Input: part model. Units: mm. Frame: model coordinates. A direction names the side the tool comes from. Round coordinates to 2 decimals unless told otherwise and drop trailing zeros. Order: outer loops, then holes, each group sorted by start corner. A loop starts at its lowest first (then second) coordinate and runs counter-clockwise, first axis right, second up.
Item 1: Cut plane A-A on z = 0. Give the number of separate pieces and of enclosed holes in the cut face, then the cut area to 3 significant figures.
Item 2: Cut plane C-C on x = 155. Output: boundary loops of the cut face in (y, z).
Item 3: Cut plane B-B on y = 0.1. Output: boundary loops of the cut face in (x, z), then the cut area to 3 significant figures.
Item 4: Cut plane D-D on x = 27. Output: boundary loops of the cut face in (y, z), then the cut area to 3 significant figures.
Item 5: Reachability of faces 1 (the flat face through (196.5, -2, 0)), 2 (the flat face through (97, -1.5, 0)) from +Z, -Z, +X, -X, +Y, -Y: full face, straight path, thin tool, end or side. Return the list, or none.
Item 6: Line query: L1, parallel to X at y = -2.3, z = 0; L2, parallel to Z at x = 54.5, y = -1.15; L3, parallel to Y at x = 139.5, z = 0.75. Output: solid intervals per line, ascending.
Item 7: Mould query, pull axis Z, two halves, no side actions, for faces 3 (the flat face through (97, 0, 5)), 4 (the flat face through (97, 2.5, 0)), 5 (the cylindrical face through (187.885, -1.993, -0.751)). Classes: released by +Z, released by -Z, zero draft, split by the parting line, or undercut.
Item 8: First-contact query: pin 1 (4 mm diameter, centred on x = 185.5, z = 0, fed in from +Y). Flat tip, straight axial feed; report the tip coordinate or a pass-through.
```python
from build123d import *

# Parameters (mm, degrees)
CROQUIS1_W              = 10
CROQUIS1_H              = 5
CROQUIS1_W_2            = 8
CROQUIS1_H_2            = 3
SALIENTE_EXTRUIR1_DEPTH = 393
CROQUIS2_R              = 2.5
CORTAR_EXTRUIR1_DEPTH   = 5
SKETCH1_W               = 196.5
SKETCH1_H               = 5
CUT_EXTRUDE1_DEPTH      = 10


with BuildPart() as part:
    # Croquis1 → Saliente-Extruir1 (new body)
    with BuildSketch(Plane(origin=(0, 0, 0), x_dir=(0, 0, -1), z_dir=(1, 0, 0))):
        Rectangle(CROQUIS1_W, CROQUIS1_H)
        Rectangle(CROQUIS1_W_2, CROQUIS1_H_2, mode=Mode.SUBTRACT)
    extrude(amount=SALIENTE_EXTRUIR1_DEPTH)

    # Croquis2 → Cortar-Extruir1 (cut)
    with BuildSketch(Plane(origin=(0, 2.5, 0), x_dir=(1, 0, 0), z_dir=(0, 1, 0))):
        with Locations((5, 0)):
            Circle(CROQUIS2_R)
        with Locations((388, 0)):
            Circle(CROQUIS2_R)
        with Locations((27, 0)):
            Circle(CROQUIS2_R)
        with Locations((366, 0)):
            Circle(CROQUIS2_R)
        with Locations((207.5, 0)):
            Circle(CROQUIS2_R)
        with Locations((185.5, 0)):
            Circle(CROQUIS2_R)
    extrude(amount=-CORTAR_EXTRUIR1_DEPTH, mode=Mode.SUBTRACT)

    # Sketch1 → Cut-Extrude1 (cut)
    with BuildSketch(Plane.XY.offset(5)):
        with Locations((294.75, 0)):
            Rectangle(SKETCH1_W, SKETCH1_H)
    extrude(amount=-CUT_EXTRUDE1_DEPTH, mode=Mode.SUBTRACT)


solid = part.part
```
From the geometry:
1. separate pieces: 8
1. enclosed holes: 0
1. area: 363 mm2
2. outline: (-2.5, -5) - (2.5, -5) - (2.5, 5) - (-2.5, 5) - close; hole (-1.5, -4) - (1.5, -4) - (1.5, 4) - (-1.5, 4) - close
3. outline: (0, -5) - (196.5, -5) - (196.5, -4) - (0, -4) - close; (0, 4) - (196.5, 4) - (196.5, 5) - (0, 5) - close
3. area: 393 mm2
4. outline: (-2.5, -5) - (2.5, -5) - (2.5, -2.5) - (1.5, -2.5) - (1.5, -4) - (-1.5, -4) - (-1.5, -2.5) - (-2.5, -2.5) - close; (-2.5, 2.5) - (-1.5, 2.5) - (-1.5, 4) - (1.5, 4) - (1.5, 2.5) - (2.5, 2.5) - (2.5, 5) - (-2.5, 5) - close
4. area: 16.0 mm2
5. face 1: +Z, -Z, +X, +Y, -Y
5. face 2: +X, -X
6. L1: x = 0 to 2.5, 7.5 to 24.5, 29.5 to 183, 188 to 196.5
6. L2: z = -5 to -4, 4 to 5
6. L3: y = -2.5 to -1.5, 1.5 to 2.5
7. face 3: released by +Z
7. face 4: zero draft
7. face 5: undercut
8. pin 1: passes through
